Part print with two shaded views. Sizes in mm from the minimum x, y, z corner. Coordinates: 2 decimals unless noted, no trailing zeros. Loops run counter-clockwise (first coordinate to the right, second up) from the corner with the lowest first, then second, coordinate; pieces in that order, holes last. Notation, with made-up numbers: (77, -35.5) - (90, -35.5) arc R16 cw to (90, -26.5) - close; hole circle Ø9 at (24.25, -8). An arc over 180 degrees is marked (long way). Write each question's results on one line, items separated by ' | '. Start each with the question number.
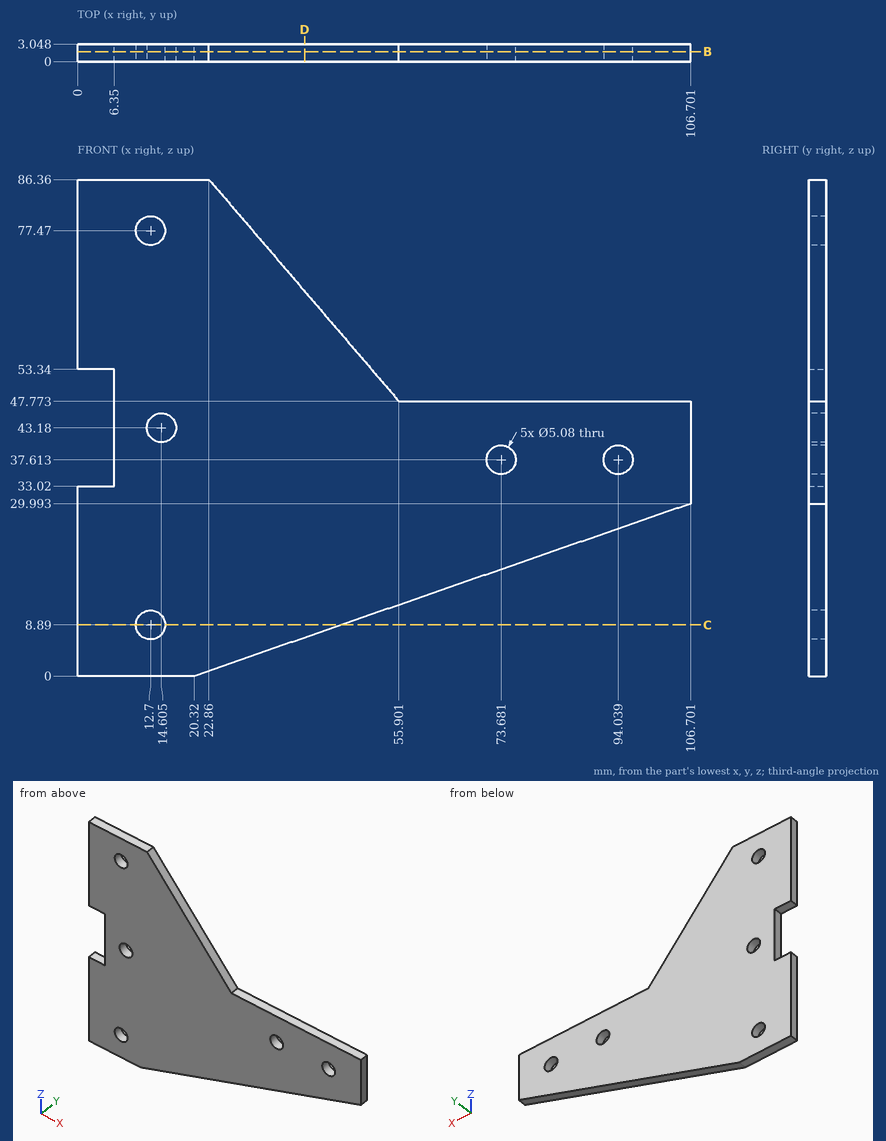
Q1. Cut at B-B (y = 1.7). State how many separate pieces and enclosed holes the cut face has, and give its area (3 significant figures).
Q2. Cut at C-C (z = 8.89). List the corners of the cut face in (x, y).
Q3. Cut at D-D (x = 39.5). List the corners of the cut face in (y, z), and give its area (3 significant figures).
Q4. Pin check, flat tips, straight feed: pin 1 (1.5 mm diameter, centred on y = 1, z = 46, fed in from -X); pin 2 (6 mm diameter, centred on x = 87, z = 18.5, fed in from +Y); pin 3 (1.5 mm diameter, centred on x = 93.5, y = 1, fed in from +Z). Stop position of each tip, or through.
Q5. Drill centre lines: L1, parallel to Z at x = 12.7, y = 1.35; L2, parallel to Z at x = 72, y = 0.7 (1 decimal); L3, parallel to X at y = 1.1, z = 59. Where is each one in solid material? Low to high. Write a range as from..to.
Check result:
1) separate pieces: 1 | enclosed holes: 5 | area: 5,090 mm²
2) outline: (0, 0) - (10.16, 0) - (10.16, 3.05) - (0, 3.05) - close; (15.24, 0) - (45.92, 0) - (45.92, 3.05) - (15.24, 3.05) - close
3) outline: (0, 6.66) - (3.05, 6.66) - (3.05, 66.93) - (0, 66.93) - close | area: 184 mm²
4) pin 1: x = 6.35 | pin 2: through | pin 3: z = 47.77
5) L1: 0..6.35, 11.43..41.5, 44.86..74.93, 80.01..86.36 | L2: 17.9..35.7, 39.5..47.8 | L3: 0..46.29
